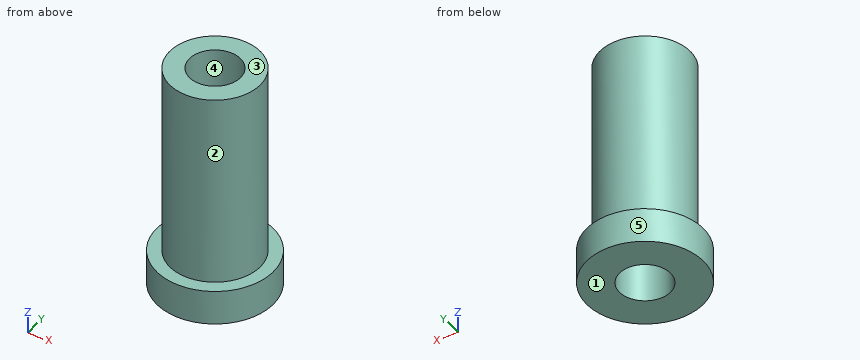
```python
from build123d import *

# Parameters (mm, degrees)
F0_R     = 5.616207
F1_DEPTH = 28.448
F2_R     = 7.235585
F3_DEPTH = 4.318
F5_D     = 6.35


with BuildPart() as f1:
    # F0 (on Top) → F1 (new body)
    with BuildSketch(Plane.XY):
        Circle(F0_R)
    extrude(amount=F1_DEPTH)

    # F2 (on Top) → F3 (join)
    with BuildSketch(Plane.XY):
        Circle(F2_R)
    extrude(amount=F3_DEPTH)

    # F5 (through all)
    with Locations(Plane(origin=(0, 0, 0), x_dir=(1, 0, 0), z_dir=(0, 0, -1))):
        with Locations((0, 0)):
            Hole(F5_D / 2)


solid = f1.part
```
Work out the finished part from the listing and answer in its coordinate system (mm). Face numbers are marked on the shaded views. A direction names the side the tool comes from. Coordinates: 2 decimals unless noted, no trailing zeros. Write each loop counter-clockwise with the first axis right and the second up, starting at its lowest first coordinate (ties: lowest second). Pieces come first, ordered by that corner, then holes. Notation, with made-up numbers: (28.25, 56) - (40.25, 56) arc R21 ccw to (40.25, 67) - close; hole circle Ø10 at (-17, 1). An arc over 180 degrees is marked (long way). Answer as a JSON object with one key per item and string values.
Q1. For a pull along Y with two mould halves and no side action, classify the marked faces 3, 4 and 5 as pulls with the +Y half, pulls with the -Y half, needs draft (parallel to the pull), parting line crosses it, or undercut.
Results list:
{"face 3": "needs draft", "face 4": "undercut", "face 5": "parting line crosses it"}
Q2. Find section D-D (y = 5.25). Write down the section's boundary in (x, z), plus the area to 3 significant figures.
Results list:
{"outline": "(-4.98, 0) - (4.98, 0) - (4.98, 4.32) - (1.99, 4.32) - (1.99, 28.45) - (-1.99, 28.45) - (-1.99, 4.32) - (-4.98, 4.32) - close", "area": "139 mm^2"}
Q3. Which of the six approach directions +Z, -Z, +X, -X, +Y, -Y give full straight-line access (tool end or side, diameter ignored) to the marked faces 1 and 2?
Results list:
{"face 1": "-Z, +X, -X, +Y, -Y", "face 2": "+Z"}
Q4. Consider L1, parallel to Y at x = 0, z = 16.5 (3 decimals); L2, parallel to Z at x = -1.25, y = -6; L3, parallel to Y at x = -0.75, z = 20.25. Determine where each line is inside the solid, lowest interval first. Write a range as from..to.
Results list:
{"L1": "y = -5.616..-3.175, 3.175..5.616", "L2": "z = 0..4.32", "L3": "y = -5.57..-3.09, 3.09..5.57"}
Q5. Given pin 1 Ø4 at (x, z) = (2.5, 17) entering from +Y; pin 2 Ø1.5 at (x, y) = (5, -1) entering from -Z; pin 3 Ø1.5 at (y, z) = (-2, 19.5) entering from -X; pin 4 Ø5.5 at (x, y) = (0, 0) entering from -Z, each flat-ended and moving along its own axis, determine where each tip first touches the part or whether it passes through.
Results list:
{"pin 1": "stops at y = 5.59", "pin 2": "stops at z = 0", "pin 3": "stops at x = -5.48", "pin 4": "passes through"}
Q6. Find section C-C (z = 26.75). Write down the section's boundary in (x, y) (3 decimals), plus the area to 3 significant figures.
Results list:
{"outline": "circle Ø11.232 at (0, 0); hole circle Ø6.35 at (0, 0)", "area": "67.4 mm^2"}
Q7. Find section A-A (x = 0). Write down the section's boundary in (y, z) (3 decimals), plus the area to 3 significant figures.
Results list:
{"outline": "(-7.236, 0) - (-3.175, 0) - (-3.175, 28.448) - (-5.616, 28.448) - (-5.616, 4.318) - (-7.236, 4.318) - close; (3.175, 0) - (7.236, 0) - (7.236, 4.318) - (5.616, 4.318) - (5.616, 28.448) - (3.175, 28.448) - close", "area": "153 mm^2"}
